Print and shaded views of the part. All mm, measured from the part's lowest x, y and z. A direction names the side the tool comes from. Round coordinates to 2 decimals unless told otherwise and drop trailing zeros. Order: outer loops, then holes, each group sorted by start corner. A loop starts at its lowest first (then second) coordinate and runs counter-clockwise, first axis right, second up. Notation, with made-up numbers: M 74,86.25 L 101,86.25 A22 ccw 101,121.25 Z; hole C 82.25,-8.5 d8. An arc over 180 degrees is marked long. Use CSV: the item, a comma, the result in double quotes.
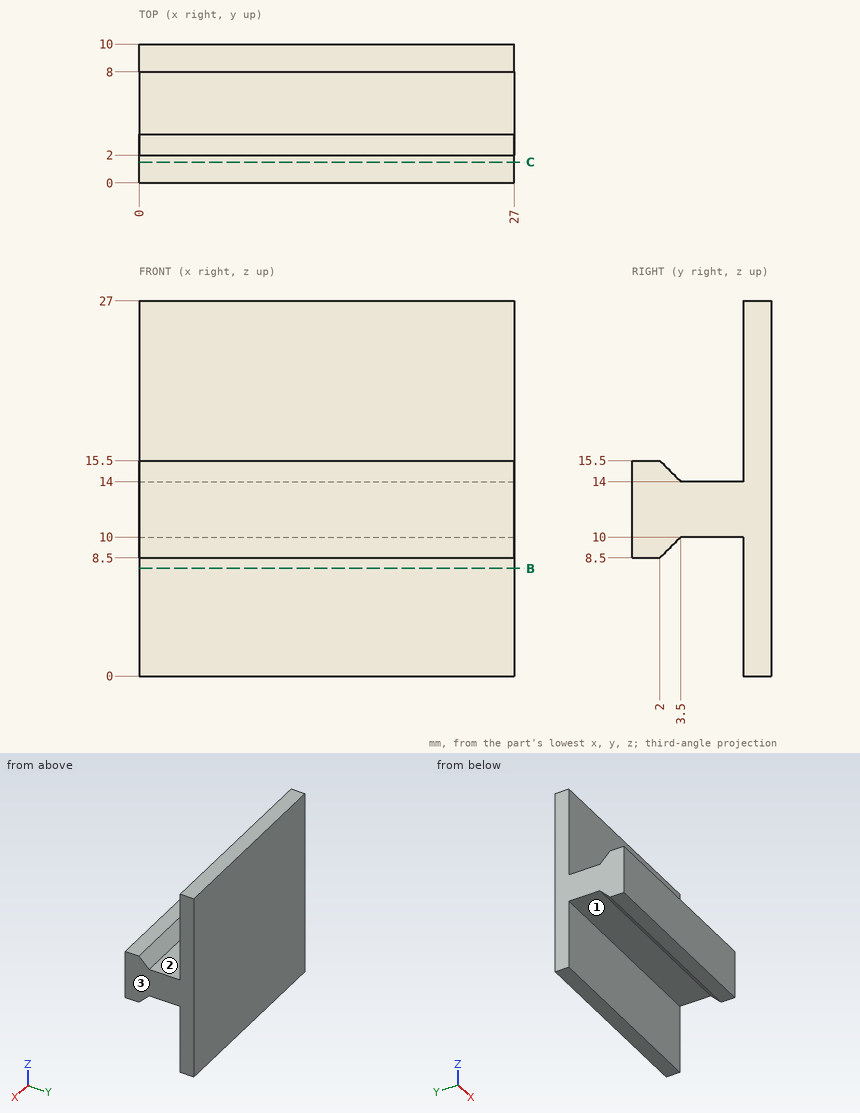
(1) Drop flat-ended pins along their axis: pin 1 (1 mm diameter, centred on x = 13, y = 1, fed in from +Z); pin 2 (6.5 mm diameter, centred on x = 16, z = 23, fed in from -Y); pin 3 (2 mm diameter, centred on x = 20, y = 1, fed in from -Z); pin 4 (5 mm diameter, centred on x = 9, z = 13, fed in from -Y). Give the stop position or say it passes through.
Answer block:
pin 1,"stops at z = 15.5"
pin 2,"stops at y = 8"
pin 3,"stops at z = 8.5"
pin 4,"stops at y = 0"
(2) Cut at C-C, the plane y = 1.5. Give the cut face in (x, z).
Answer block:
outline,"M 0,8.5 L 27,8.5 L 27,15.5 L 0,15.5 Z"
(3) Tool access for the marked faces 1, 2 and 3: list every direction of +Z, -Z, +X, -X, +Y, -Y with a clear straight run to the whole face (end or side of a thin tool).
Answer block:
face 1,"-Z, +X, -X"
face 2,"+Z, +X, -X"
face 3,"+Z, -Z, +X, +Y, -Y"
(4) Cut at B-B, the plane z = 7.75. Give the cut face in (x, y).
Answer block:
outline,"M 0,8 L 27,8 L 27,10 L 0,10 Z"
(5) Wall check: line 1 (Y direction, x = 4.25, z = 21.5); line 2 (Z direction, x = 24.25, y = 5); line 3 (Z direction, x = 23.5, y = 1). Give the ranges that are in metal, low to high. Write a range as from..to.
Answer block:
line 1,"y = 8..10"
line 2,"z = 10..14"
line 3,"z = 8.5..15.5"
